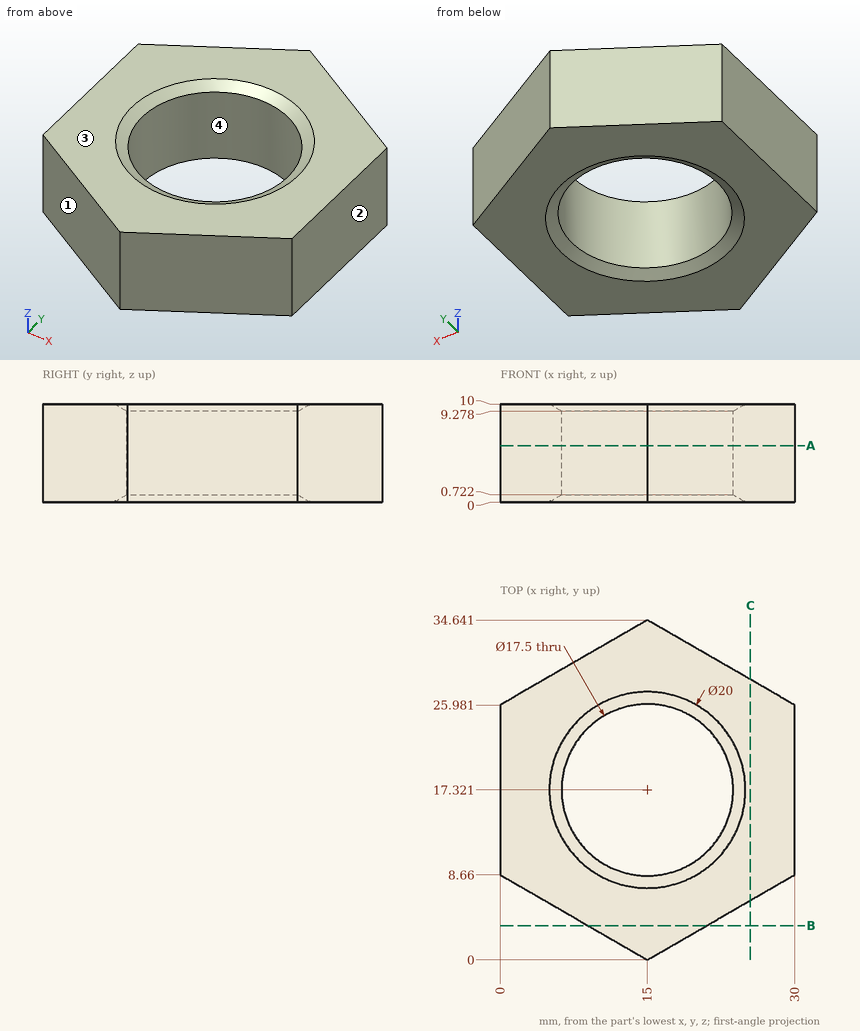
For this review, use the dimensioned drawing (mm, ordinates from the lowest corner) and the shaded views. Coordinates: 2 decimals unless noted, no trailing zeros. Loops run counter-clockwise (first coordinate to the right, second up) from the corner with the lowest first, then second, coordinate; pieces in that order, holes last. Notation, with made-up numbers: (31.25, -10.5) -> (75.25, -10.5) arc R18 cw to (75.25, 13.5) -> close; hole circle Ø6 at (55, 64.25). An arc over 180 degrees is marked (long way). Write each question's results on one line, items separated by ' | '.
Q1. Add section C-C, the plane x = 25.5. State the section outline as (y, z) points.
Taken from the geometry:
outline: (6.06, 0) -> (28.58, 0) -> (28.58, 10) -> (6.06, 10) -> close
Q2. Add section B-B, the plane y = 3.5. State the section outline as (x, z) points.
Taken from the geometry:
outline: (8.94, 0) -> (21.06, 0) -> (21.06, 10) -> (8.94, 10) -> close
Q3. To check wall thickness, follow line 1 along X through (y, z) = (10.5, 2.5); line 2 along Y through (x, z) = (9.5, 1) (1 decimal); line 3 along X through (y, z) = (20, 4.25). State the ranges of each line that lie inside material, in increasing order. Write a range as [from, to].
Taken from the geometry:
line 1: [0, 9.52], [20.48, 30] | line 2: [3.2, 10.5], [24.1, 31.5] | line 3: [0, 6.67], [23.33, 30]
Q4. Mouldability with a two-part tool opening along X and no side actions: class the marked faces 1, 2, 3 and 4 as +X half, -X half, draft (parallel to the pull), parting line (faces both ways), or undercut.
Taken from the geometry:
face 1: -X half | face 2: +X half | face 3: draft | face 4: undercut
Q5. Add section A-A, the plane z = 5.75. State the section outline as (x, y) points, then the cut area to 3 significant figures.
Taken from the geometry:
outline: (0, 8.66) -> (15, 0) -> (30, 8.66) -> (30, 25.98) -> (15, 34.64) -> (0, 25.98) -> close; hole circle Ø17.5 at (15, 17.32) | area: 539 mm²
Q6. For pin 1 Ø2 at (x, y) = (10, 21.5) entering from +Z; pin 2 Ø5 at (y, z) = (29.5, 2.5) entering from -X (1 decimal), all flat-tipped, find the tip position at first contact; note any pin that passes through.
Taken from the geometry:
pin 1: through | pin 2: x = 1.8
